Read the model definition and answer for the solid it produces. Units are mm, in the model's axes. A direction names the side the tool comes from. Coordinates: 2 decimals unless noted, no trailing zeros. Order: outer loops, then holes, each group sorted by start corner. A loop starts at its lowest first (then second) coordinate and runs counter-clockwise, first axis right, second up. Notation, with made-up numbers: (-19.5, 53.25) -> (-12.5, 53.25) arc R24 ccw to (-12.5, 69.25) -> close; hole circle Ø4 at (9, -27.5). An arc over 180 degrees is marked (long way). Use CSV: the item, a comma, the result in double quotes.
Autodesk Inventor part; units mm, degrees
ref_plane "Work Plane1" through (0, 0, 4) normal (0, 0, 1) x (1, 0, 0)
ref_plane "Work Plane3" through (0, 0, 0) normal (0, 0, 1) x (1, 0, 0)
ref_plane "Work Plane4" through (0, 0, 0) normal (0, 0, -1) x (-1, 0, 0)
sketch "Sketch1" plane through (0, 0, 0) normal (0, 0, 1) x (1, 0, 0)
  circle A0 centre (0, 0) radius 55
  dimension "d0" = 110
extrude "Extrusion1" add sketch "Sketch1" along normal blind 4
ref_plane "Work Plane1" through (0, 0, 4) normal (0, 0, 1) x (1, 0, 0)
sketch "Sketch2" plane through (0, 0, 4) normal (0, 0, 1) x (1, 0, 0)
  line L0 (-10.406, 10.152) -> (10.406, 10.152)
  line L1 (10.406, 10.152) -> (10.406, -30.726)
  line L2 (10.406, -30.726) -> (-10.406, -30.726)
  line L3 (-10.406, -30.726) -> (-10.406, 10.152)
  circle A0 centre (-35.532, 35.532) radius 1.5
  circle A1 centre (-35.532, -35.532) radius 1.5
  circle A2 centre (35.532, -35.532) radius 1.5
  circle A3 centre (35.532, 35.532) radius 1.5
  circle A4 centre (-5.08, 13.462) radius 1
  circle A5 centre (5.08, 13.462) radius 1
  circle A6 centre (-5.08, -34.036) radius 1
  circle A7 centre (5.08, -34.036) radius 1
  point P0 (0, 0)
  point P1 (0, 10.152)
  point P2 (0, -30.726)
  dimension "d78" = 30.226
  dimension "d80" = 5.08
  dimension "d82" = 5.08
  dimension "d4" = 20.812
  dimension "d5" = 40.878
  dimension "d6" = 10.152
  dimension "d7" = 3
  dimension "d8" = 3
  dimension "d9" = 3
  dimension "d10" = 3
  dimension "d11" = 2
  dimension "d12" = 2
  dimension "d13" = 2
  dimension "d14" = 2
  dimension "d15" = 35.532
  dimension "d16" = 35.532
  dimension "d17" = 35.532
  dimension "d18" = 35.532
  dimension "d19" = 35.532
  dimension "d20" = 35.532
  dimension "d21" = 35.532
  dimension "d22" = 35.532
  dimension "d23" = 10.16
  dimension "d24" = 10.16
  dimension "d25" = 3.31
  dimension "d26" = 3.31
  dimension "d27" = 3.31
  dimension "d28" = 3.31
  dimension "d47" = 30.726
  dimension "d48" = 5.08
  dimension "d49" = 5.08
  dimension "d50" = 5.08
  dimension "d51" = 5.08
  dimension "d137" = 10.152
extrude "Extrusion2" cut sketch "Sketch2" against normal blind 4 contours L0 L1 L2 L3
ref_plane "Work Plane2" through (0, 0, 4) normal (0, 0, 1) x (1, 0, 0)
sketch "Sketch3" plane through (0, 0, 4) normal (0, 0, 1) x (1, 0, 0)
  circle A0 centre (-35.577, 35.5342) radius 2.5
  circle A1 centre (-35.5225, -35.5931) radius 2.5
  circle A2 centre (35.5095, -35.5931) radius 2.5
  circle A3 centre (35.5095, 35.4262) radius 2.5
  point P0 (0, 0)
ref_plane "Work Plane3" through (0, 0, 0) normal (0, 0, 1) x (1, 0, 0)
sketch "Sketch4" plane through (0, 0, 0) normal (0, 0, 1) x (1, 0, 0)
  circle A0 centre (-35.577, 35.5342) radius 2.5
  circle A1 centre (-35.5225, -35.5931) radius 2.5
  circle A2 centre (35.5095, -35.5931) radius 2.5
  circle A3 centre (35.5095, 35.4262) radius 2.5
  point P0 (0, 0)
  point P1 (0, 0)
  dimension "d41" = 5
  dimension "d42" = 5
  dimension "d43" = 5
  dimension "d44" = 5
extrude "Extrusion3" cut sketch "Sketch4" along normal blind 0.657
ref_plane "Work Plane4" through (0, 0, 0) normal (0, 0, -1) x (-1, 0, 0)
sketch "Sketch5" plane through (0, 0, 0) normal (0, 0, -1) x (-1, 0, 0)
  line L0 (-9.906, 9.652) -> (9.906, 9.652)
  line L1 (9.906, 9.652) -> (9.906, -30.226)
  line L2 (9.906, -30.226) -> (-9.906, -30.226)
  line L3 (-9.906, -30.226) -> (-9.906, 9.652)
  circle A0 centre (-35.532, 35.532) radius 1.5
  circle A1 centre (-35.532, -35.532) radius 1.5
  circle A2 centre (35.532, -35.532) radius 1.5
  circle A3 centre (35.532, 35.532) radius 1.5
  circle A4 centre (-5.08, 13.462) radius 1
  circle A5 centre (5.08, 13.462) radius 1
  circle A6 centre (-5.08, -34.036) radius 1
  circle A7 centre (5.08, -34.036) radius 1
  point P0 (0, 0)
  point P1 (0, 0)
  point P2 (0, 9.652)
  point P3 (0, -30.226)
  dimension "d53" = 19.812
  dimension "d54" = 39.878
  dimension "d55" = 9.652
  dimension "d56" = 3
  dimension "d57" = 3
  dimension "d58" = 3
  dimension "d59" = 3
  dimension "d60" = 2
  dimension "d61" = 2
  dimension "d62" = 2
  dimension "d63" = 2
  dimension "d64" = 35.532
  dimension "d65" = 35.532
  dimension "d66" = 35.532
  dimension "d67" = 35.532
  dimension "d68" = 35.532
  dimension "d69" = 35.532
  dimension "d70" = 35.532
  dimension "d71" = 35.532
  dimension "d72" = 10.16
  dimension "d73" = 10.16
  dimension "d74" = 3.81
  dimension "d75" = 3.81
  dimension "d76" = 3.81
  dimension "d77" = 3.81
  dimension "d78" = 30.226
  dimension "d79" = 5.08
  dimension "d80" = 5.08
  dimension "d81" = 5.08
  dimension "d82" = 5.08
hole "Hole1" at (35.532, 35.532, 0) at (-35.532, 35.532, 0) at (35.532, -35.532, 0) at (-35.532, -35.532, 0) direction (0, 0, 1) diameter 2.459 depth 4 tip angle 118
ref_plane "Work Plane5" through (0, 0, 0) normal (0, 0, -1) x (-1, 0, 0)
sketch "Sketch6" plane through (0, 0, 0) normal (0, 0, -1) x (-1, 0, 0)
  line L0 (-9.906, 9.652) -> (9.906, 9.652)
  line L1 (9.906, 9.652) -> (9.906, -30.226)
  line L2 (9.906, -30.226) -> (-9.906, -30.226)
  line L3 (-9.906, -30.226) -> (-9.906, 9.652)
  circle A0 centre (-35.532, 35.532) radius 1.5
  circle A1 centre (-35.532, -35.532) radius 1.5
  circle A2 centre (35.532, -35.532) radius 1.5
  circle A3 centre (35.532, 35.532) radius 1.5
  circle A4 centre (-5.08, 13.462) radius 1
  circle A5 centre (5.08, 13.462) radius 1
  circle A6 centre (-5.08, -34.036) radius 1
  circle A7 centre (5.08, -34.036) radius 1
  point P0 (0, 0)
  point P1 (0, 0)
  point P2 (0, 0)
  point P3 (0, 9.652)
  point P4 (0, -30.226)
  dimension "d91" = 19.812
  dimension "d92" = 39.878
  dimension "d93" = 9.652
  dimension "d94" = 3
  dimension "d95" = 3
  dimension "d96" = 3
  dimension "d97" = 3
  dimension "d98" = 2
  dimension "d99" = 2
  dimension "d100" = 2
  dimension "d101" = 2
  dimension "d102" = 35.532
  dimension "d103" = 35.532
  dimension "d104" = 35.532
  dimension "d105" = 35.532
  dimension "d106" = 35.532
  dimension "d107" = 35.532
  dimension "d108" = 35.532
  dimension "d109" = 35.532
  dimension "d110" = 10.16
  dimension "d111" = 10.16
  dimension "d112" = 3.81
  dimension "d113" = 3.81
  dimension "d114" = 3.81
  dimension "d115" = 3.81
  dimension "d116" = 30.226
  dimension "d117" = 5.08
  dimension "d118" = 5.08
  dimension "d119" = 5.08
  dimension "d120" = 5.08
hole "Hole2" at (-5.08, 13.462, 0) at (5.08, 13.462, 0) at (-5.08, -34.036, 0) at (5.08, -34.036, 0) direction (0, 0, 1) diameter 1.567 depth 4 tip angle 118
fillet "Fillet1" radius 0.4125 4 edges at (10.406, -30.726, 2) (-10.406, -30.726, 2) (10.406, 10.152, 2) (-10.406, 10.152, 2)
ref_plane "Work Plane6" through (0, 0, 0) normal (0, 0, -1) x (-1, 0, 0)
sketch "Sketch7" plane through (0, 0, 0) normal (0, 0, -1) x (-1, 0, 0)
  line L0 (3.5, 12.552) -> (-3.5, 12.552)
  line L1 (-3.5, 12.552) -> (-3.5, 10.052)
  line L2 (-3.5, 10.052) -> (3.5, 10.052)
  line L3 (3.5, 10.052) -> (3.5, 12.552)
  line L4 (-9.9935, 10.152) -> (9.9935, 10.152)
  point P0 (0, 0)
  point P1 (-3.5, 10.152)
  point P2 (3.5, 10.152)
  dimension "d130" = 2.5
  dimension "d131" = 7
  dimension "d132" = 0.1
  dimension "d133" = 3.5
extrude "Extrusion4" cut sketch "Sketch7" against normal blind 4 contours L3 L4 L1 L0
fillet "Fillet2" radius 0.5 4 edges at (-3.5, 12.552, 2) (-3.5, 10.152, 2) (3.5, 12.552, 2) (3.5, 10.152, 2)
properties part number "bottom-plate_3DPrint"
Item 1: A tool of negligible diameter and unlimited length cuts with its end or side. For faces 4 (the flat face through (-7, 10.152, 2)), 5 (the flat face through (-36, 34, 0.657)), 6 (the flat face through (11, 1, 0)), from which of +Z, -Z, +X, -X, +Y, -Y can it reach the whole face along a straight path? Write none if from no direction.
Return value:
face 4,"+Z, -Z"
face 5,"-Z"
face 6,"-Z, +X, -X, +Y, -Y"
Item 2: Find section A-A, the plane x = 0. Give the vertices of the cut face in (y, z).
Return value:
outline,"(-55, 0) -> (-30.73, 0) -> (-30.73, 4) -> (-55, 4) -> close; (12.55, 0) -> (55, 0) -> (55, 4) -> (12.55, 4) -> close"
Item 3: Each of these flat-tipped pins is pushed along its axis until it touches: P1, Ø0.9, axis at x = -5.08, y = 13.462, coming from the -Z side; P2, Ø2.5, axis at x = -36.5, y = 35.5, coming from the -Z side; P3, Ø1.5, axis at x = -44, z = 1.5, coming from the +Y side; P4, Ø1.2, axis at x = -1.5, z = 3, coming from the -Y side. Where does it stop, or does it pass through?
Return value:
P1,"passes through"
P2,"stops at z = 0.66"
P3,"stops at y = 33.98"
P4,"stops at y = -54.99"
Item 4: Find section D-D, the plane x = 44.5. Give the vertices of the cut face in (y, z).
Return value:
outline,"(-32.32, 0) -> (32.32, 0) -> (32.32, 4) -> (-32.32, 4) -> close"
Item 5: Find section B-B, the plane y = 0. Give the vertices of the cut face in (x, z), then the cut area to 3 significant figures.
Return value:
outline,"(-55, 0) -> (-10.41, 0) -> (-10.41, 4) -> (-55, 4) -> close; (10.41, 0) -> (55, 0) -> (55, 4) -> (10.41, 4) -> close"
area,"357 mm^2"
Item 6: Straight lines are drawn through the part: line 1 along X through (y, z) = (-1, 3.6); line 2 along Y through (x, z) = (-8, 2); line 3 along X through (y, z) = (-3, 1.2). For each, find the intervals that lie inside material, in ascending order.
Return value:
line 1,"x = -54.99 to -10.41, 10.41 to 54.99"
line 2,"y = -54.42 to -30.73, 10.15 to 54.42"
line 3,"x = -54.92 to -10.41, 10.41 to 54.92"
Item 7: The mould has two halves that part along X. Classify faces 1 (the cylindrical face through (-11.923, 53.692, 1.972)), 2 (the flat face through (11, 1, 4)), 3 (the cylindrical face through (-33.268, 36.492, 0.324)): +X half, -X half, draft (parallel to the pull), parting line (faces both ways), or undercut.
Return value:
face 1,"parting line"
face 2,"draft"
face 3,"undercut"
Item 8: Find section C-C, the plane z = 2.85. Give the number of separate pieces and of enclosed holes in the cut face, then the cut area to 3 significant figures.
Return value:
separate pieces,"1"
enclosed holes,"9"
area,"8,610 mm^2"
